Can you work these out from the model? Positions are in its coordinate system, mm. Face numbers are marked on the shaded views. A direction names the side the tool comes from. Round coordinates to 2 decimals unless told otherwise and drop trailing zeros. Order: outer loops, then holes, each group sorted by start corner. A loop starts at its lowest first (then second) coordinate and runs counter-clockwise, first axis right, second up.
Q1. If we section it at C-C (z = -15.6): Please give me the cut outline in (x, y).
Q2. Will these pins go through, and if not, where does the flat tip stop? P1, Ø1, axis at y = 1.5, z = -5, coming from the +X side; P2, Ø4, axis at x = 8.5, z = -4.5, coming from the -Y side; P3, Ø2.5, axis at y = 1, z = 2, coming from the -X side.
Q3. If we section it at A-A (x = 23): Please give me the cut outline in (y, z), plus the area to 3 significant figures.
Q4. For the marked faces 1 and 2, which set-ups out of +Z, -Z, +X, -X, +Y, -Y let a thin tool reach every point of the face, with its end or its side?
Q5. If I drill on line 1 (Z direction, x = -26, y = 1.5); line 2 (X direction, y = 0.5, z = 8.5); line 3 (Z direction, x = 22, y = 1.5), over which ranges is the centre line in solid material (lowest first)?
Q6. If we section it at B-B (y = -8.5): Please give me the cut outline in (x, z), plus the area to 3 significant figures.
Q7. If we section it at D-D (y = 1): Please give me the cut outline in (x, z), plus the area to 3 significant figures.
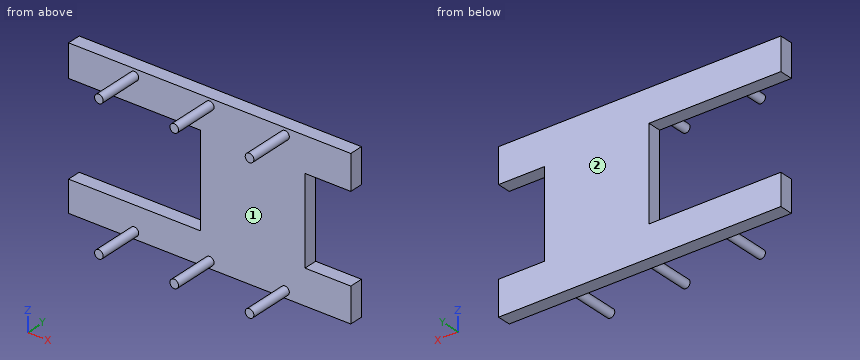
from build123d import *

# Parameters (mm, degrees)
SKETCH1_W           = 55.1
SKETCH1_H           = 27.8
BOSS_EXTRUDE1_DEPTH = 3
SKETCH3_W           = 21.65
SKETCH3_H           = 20.203759547
SKETCH3_W_2         = 17.65
SKETCH3_H_2         = 15.75
CUT_EXTRUDE1_DEPTH  = 32.00342723
SKETCH4_W           = 19.154601746
SKETCH4_H           = 20.203759547
CUT_EXTRUDE2_DEPTH  = 32.00342723
CUT_EXTRUDE3_DEPTH  = 10
SKETCH7_W           = 4.4
SKETCH7_H           = 3
BOSS_EXTRUDE2_DEPTH = 4.1
SKETCH8_W           = 3.662724417
SKETCH8_H           = 3
SKETCH8_W_2         = 3.933516036
BOSS_EXTRUDE3_DEPTH = 3
SKETCH9_W           = 62.2
SKETCH9_H           = 3
BOSS_EXTRUDE4_DEPTH = 3.21
SKETCH10_W          = 62.2
SKETCH10_H          = 3
BOSS_EXTRUDE5_DEPTH = 3.21
SKETCH11_R          = 0.95
BOSS_EXTRUDE6_DEPTH = 10


with BuildPart() as part:
    # Sketch1 → Boss-Extrude1 (new body)
    with BuildSketch(Plane(origin=(0, 0, 0), x_dir=(1, 0, 0), z_dir=(0, 1, 0))):
        Rectangle(SKETCH1_W, SKETCH1_H)
    extrude(amount=BOSS_EXTRUDE1_DEPTH)

    # Sketch3 → Cut-Extrude1 (cut, through all)
    # profile 1 of 2: a face of its own
    with BuildSketch(Plane.XZ):
        with Locations((-12.325, -0.13539581)):
            Rectangle(SKETCH3_W, SKETCH3_H)
        with Locations((-12.325, -0.375)):
            Rectangle(SKETCH3_W_2, SKETCH3_H_2, mode=Mode.SUBTRACT)
    # profile 2 of 2: a face of its own
    with BuildSketch(Plane.XZ):
        with Locations((-12.325, -0.375)):
            Rectangle(SKETCH3_W_2, SKETCH3_H_2)
    extrude(amount=-CUT_EXTRUDE1_DEPTH, mode=Mode.SUBTRACT)

    # Sketch4 → Cut-Extrude2 (cut, through all)
    with BuildSketch(Plane(origin=(0, 3, 0), x_dir=(1, 0, 0), z_dir=(0, 1, 0))):
        with Locations((-32.727300873, 0.13539581)):
            Rectangle(SKETCH4_W, SKETCH4_H)
    extrude(amount=-CUT_EXTRUDE2_DEPTH, mode=Mode.SUBTRACT)

    # Sketch5 → Cut-Extrude3 (cut)
    with BuildSketch(Plane(origin=(0, 3, 0), x_dir=(1, 0, 0), z_dir=(0, 1, 0))):
        Polygon((27.55, -9.5), (27.55, 0), (27.55, 9.5), (21.55, 9.5), (21.55, -9.5), align=None)
    extrude(amount=-CUT_EXTRUDE3_DEPTH, mode=Mode.SUBTRACT)

    # Sketch7 → Boss-Extrude2 (add)
    with BuildSketch(Plane(origin=(27.55, 0, 0), x_dir=(0, 0, -1), z_dir=(1, 0, 0))):
        with Locations((11.7, 1.5)):
            Rectangle(SKETCH7_W, SKETCH7_H)
        with Locations((-11.7, 1.5)):
            Rectangle(SKETCH7_W, SKETCH7_H)
    extrude(amount=BOSS_EXTRUDE2_DEPTH)

    # Sketch8 → Boss-Extrude3 (add)
    with BuildSketch(Plane.ZY.offset(27.55)):
        with Locations((-12.068637792, 1.5)):
            Rectangle(SKETCH8_W, SKETCH8_H)
        with Locations((11.933241982, 1.5)):
            Rectangle(SKETCH8_W_2, SKETCH8_H)
    extrude(amount=BOSS_EXTRUDE3_DEPTH)

    # Sketch9 → Boss-Extrude4 (add)
    with BuildSketch(Plane(origin=(0, 0, -13.9), x_dir=(-1, 0, 0), z_dir=(0, 0, -1))):
        with Locations((-0.55, 1.5)):
            Rectangle(SKETCH9_W, SKETCH9_H)
    extrude(amount=BOSS_EXTRUDE4_DEPTH)

    # Sketch10 → Boss-Extrude5 (add)
    with BuildSketch(Plane.XY.offset(13.9)):
        with Locations((0.55, 1.5)):
            Rectangle(SKETCH10_W, SKETCH10_H)
    extrude(amount=BOSS_EXTRUDE5_DEPTH)

    # Sketch11 → Boss-Extrude6 (add)
    with BuildSketch(Plane.XZ):
        with Locations(Location((-16.05, 15.6, 0), (0, 0, 90))):
            Circle(SKETCH11_R)
        with Locations(Location((-16.05, -15.6, 0), (0, 0, 90))):
            Circle(SKETCH11_R)
        with Locations(Location((0.55, -15.6, 0), (0, 0, 90))):
            Circle(SKETCH11_R)
        with Locations(Location((0.55, 15.6, 0), (0, 0, 90))):
            Circle(SKETCH11_R)
        with Locations(Location((17.15, 15.6, 0), (0, 0, 90))):
            Circle(SKETCH11_R)
        with Locations(Location((17.15, -15.6, 0), (0, 0, 90))):
            Circle(SKETCH11_R)
    extrude(amount=BOSS_EXTRUDE6_DEPTH)


solid = part.part
Solution:
1. outline: (-30.55, 0) - (-17, 0) - (-17, -10) - (-15.1, -10) - (-15.1, 0) - (-0.4, 0) - (-0.4, -10) - (1.5, -10) - (1.5, 0) - (16.2, 0) - (16.2, -10) - (18.1, -10) - (18.1, 0) - (31.65, 0) - (31.65, 3) - (-30.55, 3) - close
2. P1: stops at x = 21.55
2. P2: stops at y = 0
2. P3: stops at x = -1.5
3. outline: (0, -17.11) - (3, -17.11) - (3, -9.5) - (0, -9.5) - close; (0, 9.5) - (3, 9.5) - (3, 17.11) - (0, 17.11) - close
3. area: 45.7 mm2
4. face 1: -Y
4. face 2: +Z, -Z, +X, -X, +Y
5. line 1: z = -17.11 to -10.24, 9.97 to 17.11
5. line 2: x = -1.5 to 21.55
5. line 3: z = -17.11 to -9.5, 9.5 to 17.11
6. outline: circle Ø1.9 at (-16.05, -15.6); circle Ø1.9 at (-16.05, 15.6); circle Ø1.9 at (0.55, -15.6); circle Ø1.9 at (0.55, 15.6); circle Ø1.9 at (17.15, -15.6); circle Ø1.9 at (17.15, 15.6)
6. area: 17.0 mm2
7. outline: (-30.55, -17.11) - (31.65, -17.11) - (31.65, -9.5) - (21.55, -9.5) - (21.55, 9.5) - (31.65, 9.5) - (31.65, 17.11) - (-30.55, 17.11) - (-30.55, 9.97) - (-1.5, 9.97) - (-1.5, -10.24) - (-30.55, -10.24) - close
7. area: 1,350 mm2
